```python
from build123d import *

# Parameters (mm, degrees)
F0_W     = 48
F0_H     = 15
F1_DEPTH = 20
F2_R     = 4.5
F3_DEPTH = 1.5
F4_DEPTH = 19
F5_T     = -0.5


with BuildPart() as f1:
    # F0 (on Front) → F1 (new body, symmetric)
    with BuildSketch(Plane.XZ):
        with Locations((2, 7.5)):
            Rectangle(F0_W, F0_H)
    extrude(amount=F1_DEPTH, both=True)

    # F2 (on face) → F3 (join)
    with BuildSketch(Plane.YZ.offset(26)):
        Polygon((-15.6143782777, 7.5), (-9, 0), (0, 0), (9, 0), (15.6143782777, 7.5), (9, 15), (0, 15), (-9, 15), align=None)
        with Locations((0, 7.5)):
            Circle(F2_R, mode=Mode.SUBTRACT)
    extrude(amount=F3_DEPTH)

    # F4 (add): a face of the model
    f4_faces = [f1.faces().sort_by_distance(p)[0] for p in [
        (26, 0, 7.5),
    ]]
    extrude(f4_faces, amount=F4_DEPTH)

    # F5
    f5_openings = [f1.faces().sort_by_distance(p)[0] for p in [
        (45, 0, 7.5),
    ]]
    offset(amount=F5_T, openings=f5_openings, kind=Kind.INTERSECTION)


solid = f1.part
```
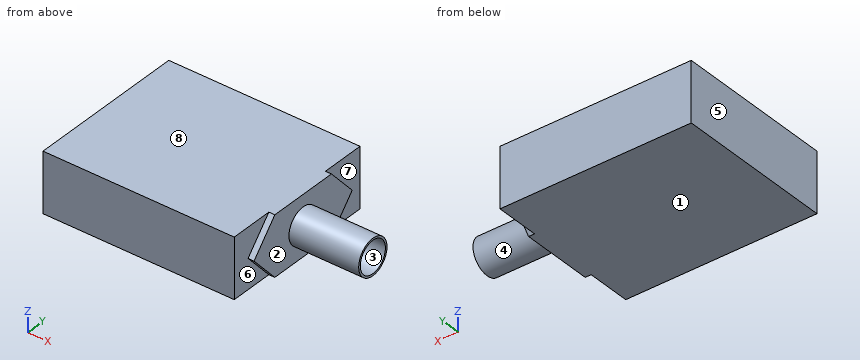
Here's how the part is built. I have some questions about the finished solid (model axes, mm). Face numbers are marked on the shaded views. A direction names the side the tool comes from. Give positions to 0.01 mm unless a question says otherwise; leave off trailing zeros. Loops run counter-clockwise (first coordinate to the right, second up) from the corner with the lowest first, then second, coordinate; pieces in that order, holes last. Notation, with made-up numbers: (-12.75, 65) -> (13.25, 65) arc R6 cw to (13.25, 73) -> close; hole circle Ø11 at (69.25, 35). An arc over 180 degrees is marked (long way). Use one line per item in the form item = value. Start each with the question number.
1) Please list where these lines run through material, in increasing order: line 1 along Y through (x, z) = (-7.5, 7.5); line 2 along X through (y, z) = (6, 8.75); line 3 along Z through (x, y) = (39, 0).
2) Imagine slicing it at A-A (y = -7). Please give me the cut outline in (x, z).
3) Imagine slicing it at B-B (x = -4). Please give me the cut outline in (y, z), then the cut area to 3 significant figures.
4) Thinking about a two-plate mould opening in Z: for the marked faces 1, 2 and 3, which applies, +Z half, -Z half, draft (parallel to the pull), parting line (faces both ways), or undercut?
5) Which directions (+Z, -Z, +X, -X, +Y, -Y) give clear straight access to the entire face, cutting with the end or side of a thin tool? Please do the marked faces 4, 5, 6, 7 and 8.
6) Imagine slicing it at D-D (z = 13.5). Please give me the cut outline in (x, y), then the cut area to 3 significant figures.
7) Imagine slicing it at C-C (y = 0). Please give me the cut outline in (x, z), then the cut area to 3 significant figures.
8) For P1, Ø3.5, axis at y = -13.5, z = 11, coming from the +X side; P2, Ø7, axis at y = 7, z = 8.5, coming from the +X side; P3, Ø3.5, axis at y = 17, z = 10, coming from the +X side, each with a flat end and sliding along its axis, tell me the tip position at first contact or that it passes through.
Check values:
q1.line_1 = -20 to -19.5, 19.5 to 20
q1.line_2 = -22 to -21.5, 27 to 27.5
q1.line_3 = 3 to 3.5, 11.5 to 12
q2.outline = (-22, 0) -> (27.5, 0) -> (27.5, 15) -> (-22, 15) -> close; hole (-21.5, 0.5) -> (27, 0.5) -> (27, 14.5) -> (-21.5, 14.5) -> close
q3.outline = (-20, 0) -> (20, 0) -> (20, 15) -> (-20, 15) -> close; hole (-19.5, 0.5) -> (19.5, 0.5) -> (19.5, 14.5) -> (-19.5, 14.5) -> close
q3.area = 54.0 mm^2
q4.face_1 = -Z half
q4.face_2 = draft
q4.face_3 = undercut
q5.face_4 = +X
q5.face_5 = +Z, -Z, -X, +Y, -Y
q5.face_6 = +X, -Y
q5.face_7 = +X, +Y
q5.face_8 = +Z, +X, -X, +Y, -Y
q6.outline = (-22, -20) -> (26, -20) -> (26, -10.32) -> (27.5, -10.32) -> (27.5, 10.32) -> (26, 10.32) -> (26, 20) -> (-22, 20) -> close; hole (-21.5, -19.5) -> (25.5, -19.5) -> (25.5, -9.66) -> (27, -9.66) -> (27, 9.66) -> (25.5, 9.66) -> (25.5, 19.5) -> (-21.5, 19.5) -> close
q6.area = 89.0 mm^2
q7.outline = (-22, 0) -> (27.5, 0) -> (27.5, 3) -> (45, 3) -> (45, 3.5) -> (27, 3.5) -> (27, 0.5) -> (-21.5, 0.5) -> (-21.5, 14.5) -> (27, 14.5) -> (27, 11.5) -> (45, 11.5) -> (45, 12) -> (27.5, 12) -> (27.5, 15) -> (-22, 15) -> close
q7.area = 77.0 mm^2
q8.P1 = 27.5
q8.P2 = 45
q8.P3 = 26
